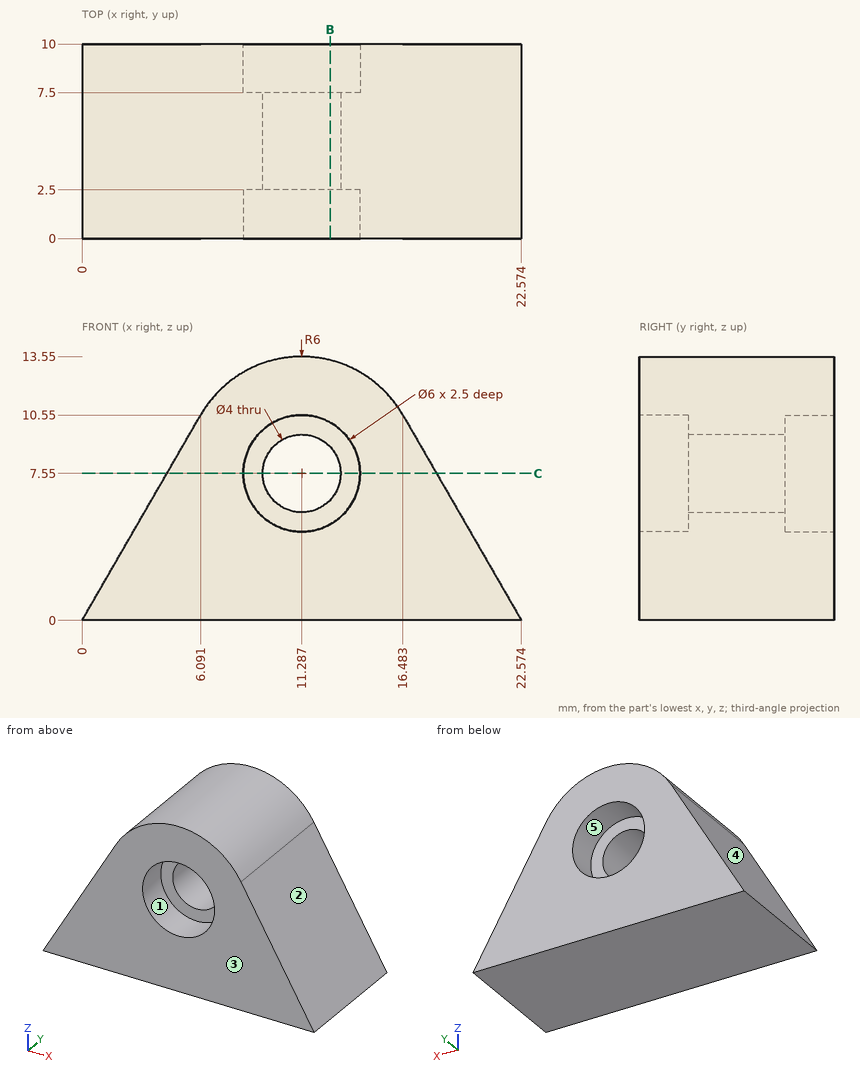
Input: dimensioned drawing with shaded views. Units: mm. Origin: part minimum x, y, z. A direction names the side the tool comes from. Round coordinates to 2 decimals unless told otherwise and drop trailing zeros. Order: outer loops, then holes, each group sorted by start corner. A loop starts at its lowest first (then second) coordinate and runs counter-clockwise, first axis right, second up. Notation, with made-up numbers: (21, -10) - (49, -10) arc R32 cw to (49, 28) - close; hole circle Ø3 at (4.5, 37.5). An arc over 180 degrees is marked (long way). Use CSV: the item, a comma, the result in double quotes. Start each with the question number.
Q1. First-contact query: pin 1 (3 mm diameter, centred on x = 15, y = 6, fed in from +Z); pin 2 (4.5 mm diameter, centred on x = 11.29, z = 7.55, fed in from +Y); pin 3 (1 mm diameter, centred on x = 4.5, y = 4, fed in from +Z). Flat tips, straight axial feed; report the tip coordinate or a pass-through.
Q2. Material intervals for line 1 along Z through (x, y) = (14, 8) (1 decimal); line 2 along X through (y, z) = (9, 5) (1 decimal); line 3 along X through (y, z) = (4.55, 7.55) (1 decimal), sorted ascending. Write a range as from..to.
Q3. Mould query, pull axis Z, two halves, no side actions, for the marked faces 1, 2 and 3. Classes: +Z half, -Z half, draft (parallel to the pull), parting line (faces both ways), or undercut.
Q4. Section query B-B (x = 12.75). Return loops of the section in (y, z).
Q5. Section query C-C (z = 7.55). Return loops of the section in (x, y) (1 decimal).
Q6. Access query for the marked faces 4 and 5. Directions: +Z, -Z, +X, -X, +Y, -Y. A direction counts if a zero-diameter tool reaches every point of the face in a straight line with its end or side. Return the directions, or none.
Result set:
1,pin 1,"stops at z = 13.13"
1,pin 2,"stops at y = 7.5"
1,pin 3,"stops at z = 8.66"
2,line 1,"z = 0..6.3, 8.8..12.9"
2,line 2,"x = 2.9..9.7, 12.9..19.7"
2,line 3,"x = 4.4..9.3, 13.3..18.2"
3,face 1,"undercut"
3,face 2,"+Z half"
3,face 3,"draft"
4,outline,"(0, 0) - (10, 0) - (10, 4.93) - (7.5, 4.93) - (7.5, 6.19) - (2.5, 6.19) - (2.5, 4.93) - (0, 4.93) - close; (0, 10.17) - (2.5, 10.17) - (2.5, 8.91) - (7.5, 8.91) - (7.5, 10.17) - (10, 10.17) - (10, 13.37) - (0, 13.37) - close"
5,outline,"(4.4, 0) - (8.3, 0) - (8.3, 2.5) - (9.3, 2.5) - (9.3, 7.5) - (8.3, 7.5) - (8.3, 10) - (4.4, 10) - close; (13.3, 2.5) - (14.3, 2.5) - (14.3, 0) - (18.2, 0) - (18.2, 10) - (14.3, 10) - (14.3, 7.5) - (13.3, 7.5) - close"
6,face 4,"+Z, -X, +Y, -Y"
6,face 5,"+Y"
